Design review of the part built by this model. Coordinates are the model's own, in mm. Coordinates: 2 decimals unless noted, no trailing zeros. Order: outer loops, then holes, each group sorted by start corner. A loop starts at its lowest first (then second) coordinate and runs counter-clockwise, first axis right, second up. Notation, with made-up numbers: M 21,80 L 42,80 A21 cw 42,107 Z; hole C 47,17 d9. An arc over 180 degrees is marked long. Answer in a Markdown table with one row per item.
Autodesk Inventor part; units mm, degrees
ref_plane "YZ Plane" through (0, 0, 0) normal (1, 0, 0) x (0, 1, 0)
ref_plane "XZ Plane" through (0, 0, 0) normal (0, 1, 0) x (-1, 0, 0)
ref_plane "XY Plane" through (0, 0, 0) normal (0, 0, 1) x (1, 0, 0)
sketch "Boceto1" plane through (0, 0, 0) normal (0, 0, 1) x (1, 0, 0)
  arc A0 (0, 5) -> (0, -5) centre (0, 0) ccw
  arc A1 (85, -5) -> (85, 5) centre (85, 0) ccw
  line L0 (0, 5) -> (85, 5)
  line L1 (0, -5) -> (85, -5)
  circle A2 centre (0, 0) radius 2.5
  circle A3 centre (85, 0) radius 2.5
  dimension "d1" = 10
  dimension "d2" = 10
  dimension "d3" = 5
  dimension "d4" = 5
  dimension "d7" = 85
extrude "Extrusión1" add sketch "Boceto1" along normal blind 5
(1) Insertion check: pin 1 Ø1.5 at (y, z) = (3, 3) entering from -X. The pin has a flat end and moves straight along its axis. Give the tip position at first contact, or say it passes through.
Return value:
| item | result |
|---|---|
| pin 1 | stops at x = -4.47 |
(2) Draft analysis for pull direction X (two halves, no side actions). For faces 1 (the flat face through (42, -5, 2)), 2 (the cylindrical face through (-0.54, 2.44, 2.46)), 3 (the cylindrical face through (90, 0, 2)), 4 (the cylindrical face through (82.5, -0.1, 2.5)), state which applies: pulls with the +X half, pulls with the -X half, needs draft (parallel to the pull), parting line crosses it, or undercut.
Return value:
| item | result |
|---|---|
| face 1 | needs draft |
| face 2 | undercut |
| face 3 | pulls with the +X half |
| face 4 | undercut |
(3) Add section A-A, the plane z = 1.15. Give the boundary of the cut face in (x, y), and give its area (3 significant figures).
Return value:
| item | result |
|---|---|
| outline | M 0,-5 L 85,-5 A5 ccw 85,5 L 0,5 A5 ccw Z; hole C 0,0 d5; hole C 85,0 d5 |
| area | 889 mm2 |
(4) For line 1 along Y through (x, z) = (85, 1.6); line 2 along X through (y, z) = (1, 1.8); line 3 along X through (y, z) = (2, 0.8), list the stretches that pass through material, from the lowest coordinate up. Write a range as from..to.
Return value:
| item | result |
|---|---|
| line 1 | y = -5..-2.5, 2.5..5 |
| line 2 | x = -4.9..-2.29, 2.29..82.71, 87.29..89.9 |
| line 3 | x = -4.58..-1.5, 1.5..83.5, 86.5..89.58 |
